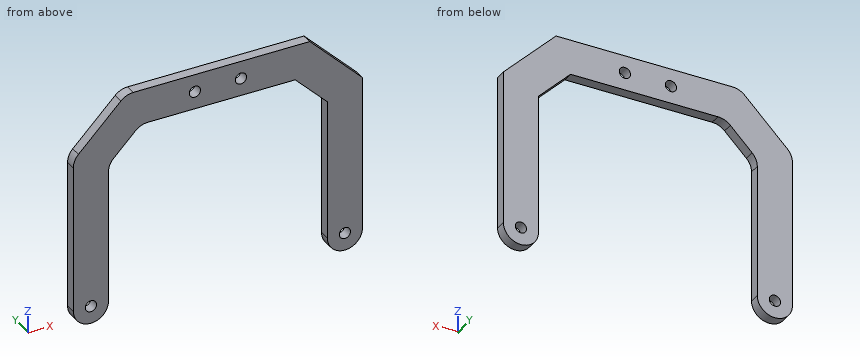
Autodesk Inventor part; units mm, degrees
ref_plane "YZ Plane" through (0, 0, 0) normal (1, 0, 0) x (0, 1, 0)
ref_plane "XZ Plane" through (0, 0, 0) normal (0, 1, 0) x (-1, 0, 0)
ref_plane "XY Plane" through (0, 0, 0) normal (0, 0, 1) x (1, 0, 0)
sketch "Sketch3" plane through (0, 0, 0) normal (0, 1, 0) x (-1, 0, 0)
  line L0 (0, 0) -> (22, 0)
  line L1 (31.1421, -9.1421) -> (31.1421, -49.1421)
  line L2 (41.1421, -49.1421) -> (41.1421, -5)
  line L3 (0, 10) -> (0, 0)
  line L4 (26.1421, 10) -> (41.1421, -5)
  line L5 (31.1421, -9.1421) -> (22, 0)
  line L6 (26.1421, 10) -> (0, 10)
  line L7 (22, 0) -> (0, 0)
  line L8 (31.1421, -9.1421) -> (31.1421, -49.1421)
  line L9 (41.1421, -49.1421) -> (41.1421, -5)
  line L10 (22, 0) -> (0, 0)
  arc A0 (31.1421, -49.1421) -> (41.1421, -49.1421) centre (36.1421, -49.1421) ccw
  circle A1 centre (0, -30) radius 30
  point P0 (31.1421, -29.1421)
  dimension "d51" = 10
  dimension "d56" = 10
  dimension "d57" = 15
  dimension "d58" = 15
  dimension "d59" = 5
  dimension "d60" = 22
  dimension "d61" = 40
  dimension "d64" = 10
  dimension "d65" = 10
  dimension "d66" = 60
  dimension "d67" = 30
extrude "Extrusion2" add sketch "Sketch3" along normal blind 3 contours L3 L6 L4 L2 A0 L1 L5 L0
sketch "Sketch4" plane through (0, 3, 0) normal (0, 1, 0) x (1, 0, 0)
  line L0 (0, -10) -> (0, 0)
  arc A0 (-31.1421, 49.1421) -> (-41.1421, 49.1421) centre (-36.1421, 49.1421) ccw
  point P0 (-6.55, -5)
  point P1 (0, -5)
  point P2 (-36.1421, 54.1421)
  dimension "d77" = 6.55
hole "Hole2" at (-6.55, 3, 5) at (-36.1421, 3, -49.1421) direction (0, -1, 0) diameter 3.2 end through all
fillet "Fillet1" radius 5 4 edges at (-26.1421, 1.5, 10) (-41.1421, 1.5, -5) (-31.1421, 1.5, -9.1421) (-22, 1.5, 0)
mirror "Mirror3" about plane through (0, 0, 10) normal (1, 0, 0) of "Extrusion2", "Hole2"
properties part number "Claw4" material "Copper, Cast"
Model file for the job. Use its own axes, mm. Coordinates: 2 decimals unless noted, no trailing zeros. Order: outer loops, then holes, each group sorted by start corner. A loop starts at its lowest first (then second) coordinate and runs counter-clockwise, first axis right, second up. Notation, with made-up numbers: (71.5, 51) - (118.5, 51) arc R7 ccw to (118.5, 58) - close; hole circle Ø3 at (5, 73). An arc over 180 degrees is marked (long way). Return JSON: item names as keys, results as strings. Group by question number.
1) Probe line 1 (X direction, y = 1.15, z = 5); line 2 (Z direction, x = 6.55, y = 2.15); line 3 (X direction, y = 0.3, z = -41). List the from-to ranges inside material, lowest first. Write a range as from..to.
2) Saw through at B-B, the plane z = -32.5. Write the cut outline in (x, y), plus the area to 3 significant figures.
3) Saw through at C-C, the plane x = 6.55. Write the cut outline in (y, z).
4) Saw through at A-A, the plane z = 5. Write the cut outline in (x, y), plus the area to 3 significant figures.
5) Saw through at D-D, the plane y = 2.4. Write the cut outline in (x, z), plus the area to 3 significant figures.
Values found:
{
 "1": {"line 1": "x = -31.14..-8.15, -4.95..4.95, 8.15..31.14", "line 2": "z = 0..3.4, 6.6..10", "line 3": "x = -41.14..-31.14, 31.14..41.14"},
 "2": {"outline": "(-41.14, 0) - (-31.14, 0) - (-31.14, 3) - (-41.14, 3) - close; (31.14, 0) - (41.14, 0) - (41.14, 3) - (31.14, 3) - close", "area": "60.0 mm²"},
 "3": {"outline": "(0, 0) - (3, 0) - (3, 3.4) - (0, 3.4) - close; (0, 6.6) - (3, 6.6) - (3, 10) - (0, 10) - close"},
 "4": {"outline": "(-31.14, 0) - (-8.15, 0) - (-8.15, 3) - (-31.14, 3) - close; (-4.95, 0) - (4.95, 0) - (4.95, 3) - (-4.95, 3) - close; (8.15, 0) - (31.14, 0) - (31.14, 3) - (8.15, 3) - close", "area": "168 mm²"},
 "5": {"outline": "(-41.14, -49.14) arc R5 ccw to (-31.14, -49.14) - (-31.14, -11.21) arc R5 cw to (-29.68, -7.68) - (-23.46, -1.46) arc R5 cw to (-19.93, 0) - (22, 0) - (31.14, -9.14) - (31.14, -49.14) arc R5 ccw to (41.14, -49.14) - (41.14, -5) - (26.14, 10) - (-24.07, 10) arc R5 ccw to (-27.61, 8.54) - (-39.68, -3.54) arc R5 ccw to (-41.14, -7.07) - close; hole circle Ø3.2 at (-36.14, -49.14); hole circle Ø3.2 at (-6.55, 5); hole circle Ø3.2 at (6.55, 5); hole circle Ø3.2 at (36.14, -49.14)", "area": "1,710 mm²"}
}
